Autodesk Inventor part; units mm, degrees
ref_plane "YZ Plane" through (0, 0, 0) normal (1, 0, 0) x (0, 1, 0)
ref_plane "XZ Plane" through (0, 0, 0) normal (0, 1, 0) x (-1, 0, 0)
ref_plane "XY Plane" through (0, 0, 0) normal (0, 0, 1) x (1, 0, 0)
sketch "Sketch1" plane through (0, 0, 0) normal (0, 1, 0) x (-1, 0, 0)
  line L0 (0, 0) -> (73, 0)
  line L1 (73, 0) -> (73, -56)
  line L2 (73, -56) -> (0, -56)
  line L3 (0, -56) -> (0, 0)
  dimension "d0" = 73
  dimension "d1" = 56
extrude "Extrusion1" add sketch "Sketch1" along normal blind 5
sketch "Sketch2" plane through (0, 5, 0) normal (0, 1, 0) x (1, 0, 0)
  line L0 (-73, 46) -> (-63, 46)
  line L1 (-63, 46) -> (-63, 36)
  line L2 (-63, 36) -> (-73, 36)
  line L3 (-73, 36) -> (-73, 46)
  line L4 (-10, 46) -> (0, 46)
  line L5 (0, 46) -> (0, 36)
  line L6 (0, 36) -> (-10, 36)
  line L7 (-10, 36) -> (-10, 46)
  line L8 (-73, 20) -> (-63, 20)
  line L9 (-63, 20) -> (-63, 10)
  line L10 (-63, 10) -> (-73, 10)
  line L11 (-73, 10) -> (-73, 20)
  line L12 (-10, 20) -> (0, 20)
  line L13 (0, 20) -> (0, 10)
  line L14 (0, 10) -> (-10, 10)
  line L15 (-10, 10) -> (-10, 20)
  line L16 (-73, 56) -> (-73, 0)
  line L17 (0, 0) -> (0, 56)
  line L18 (0, 56) -> (-73, 56)
  line L19 (-73, 0) -> (0, 0)
  dimension "d4" = 10
  dimension "d5" = 10
  dimension "d6" = 10
  dimension "d7" = 10
  dimension "d8" = 10
  dimension "d9" = 10
  dimension "d10" = 10
  dimension "d11" = 10
  dimension "d12" = 10
  dimension "d13" = 10
  dimension "d14" = 10
  dimension "d15" = 10
extrude "Extrusion2" add sketch "Sketch2" along normal blind 10 contours L0 L1 L2 L3 | L8 L9 L10 L11 | L5 L6 L7 L4 | L13 L14 L15 L12
hole "Hole1" at (-68, 10, -46) direction (0, 0, 1) diameter 4.3 end through all
hole "Hole2" at (-5, 10, -46) direction (0, 0, 1) diameter 4.3 end through all
sketch "Sketch4" plane through (0, 0, 0) normal (0, -1, 0) x (1, 0, 0)
  line L0 (-63.15, 19.6) -> (-9.85, 19.6)
  line L1 (-9.85, 19.6) -> (-9.85, -49)
  line L2 (-9.85, -49) -> (-63.15, -49)
  line L3 (-63.15, -49) -> (-63.15, 19.6)
  line L4 (0, -56) -> (-73, -56)
  line L5 (-73, 0) -> (-73, -56)
  circle A0 centre (-55.55, -46.5) radius 1.6
  circle A1 centre (-27.65, -46.5) radius 1.6
  circle A2 centre (-12.45, 4.3) radius 1.6
  circle A3 centre (-60.65, 5.6) radius 1.6
  point P0 (0, 0)
  dimension "d40" = 53.3
  dimension "d41" = 68.6
  dimension "d42" = 7
  dimension "d43" = 9.85
  dimension "d44" = 3.2
  dimension "d45" = 3.2
  dimension "d46" = 3.2
  dimension "d47" = 3.2
  dimension "d48" = 14
  dimension "d49" = 15.3
  dimension "d50" = 2.5
  dimension "d51" = 7.6
  dimension "d52" = 66.1
  dimension "d53" = 66.1
  dimension "d54" = 27.9
  dimension "d55" = 15.2
sketch "Sketch5" plane through (-73, 0, 0) normal (0, 0, 1) x (1, 0, 0)
  line L0 (10, 5) -> (63, 5)
  line L1 (63, 5) -> (63, 0)
  line L2 (63, 0) -> (10, 0)
  line L3 (10, 0) -> (10, 5)
  line L4 (73, 0) -> (0, 0)
  line L5 (0, 5) -> (73, 5)
  line L6 (73, 0) -> (73, 5)
  dimension "d56" = 10
  dimension "d57" = 10
extrude "Extrusion3" add sketch "Sketch5" along normal blind 10 contours L0 L1 L2 L3
extrude "Extrusion4" cut sketch "Sketch4" against normal up to next contours A0 | A1 | A2 | A3
properties part number "arduinoPlate" material "ABS Plastic"
The model under review builds one solid part; all positions refer to its coordinate system, in mm. A direction names the side the tool comes from. Round coordinates to 2 decimals unless told otherwise and drop trailing zeros. Write each loop counter-clockwise with the first axis right and the second up, starting at its lowest first coordinate (ties: lowest second). Pieces come first, ordered by that corner, then holes. Notation, with made-up numbers: M 4,55 L 14,55 A29 cw 14,88 Z; hole C -12.5,-20 d7. An arc over 180 degrees is marked long. Use a Markdown table: item, result. Add a question column.
Q1. We need section D-D, the plane z = 1.5. State the section outline as (x, y) points, plus the area to 3 significant figures.
Q2. To check wall thickness, follow line 1 (X direction, y = 10, z = -42.5); line 2 (Y direction, x = -68, z = -39.5); line 3 (X direction, y = 7.75, z = -15). State the ranges of each line that lie inside material, in increasing order.
Q3. We need section C-C, the plane y = 11.25. Count the separate pieces of the cut face and the enclosed holes in it, plus the area to 3 significant figures.
Q4. Machinability: for faces 4 (the face through (-65.7, 9.9, -36)), 5 (the face through (-65.7, 9.9, -10)), 6 (the face through (-63, 10, -41)), 7 (the face through (-63, 2, 5)), 8 (the face through (-5, 2, 0)), which of the approach directions +Z, -Z, +X, -X, +Y, -Y give a long, thin tool a straight path to every point of the face, cutting with its end or side? Answer none if there is none.
Q5. Insertion check: pin 1 (5 mm diameter, centred on x = -69.5, y = 9, fed in from -Z); pin 2 (4 mm diameter, centred on x = -12.45, z = 4.3, fed in from +Y); pin 3 (1.5 mm diameter, centred on y = 3, z = 4, fed in from -X). Each pin has a flat end and moves straight along its axis. Give the tip position at first contact, or say it passes through.
Q6. We need section B-B, the plane x = -5. State the section outline as (y, z) points, plus the area to 3 significant figures.
Q7. We need section A-A, the plane x = -12.45. State the section outline as (y, z) points.
Q8. The part is to be moulded in two halves that separate along Y. For faces 1 (the face through (-66.09, 10.99, -14.93)), 2 (the face through (-37, 3, 10)), 3 (the face through (-5, 15, -15)), say which applies: pulls with the +Y half, pulls with the -Y half, needs draft (parallel to the pull), parting line crosses it, or undercut.
Findings below:
| question | item | result |
|---|---|---|
| 1 | outline | M -63,0 L -10,0 L -10,5 L -63,5 Z |
| 1 | area | 265 mm² |
| 2 | line 1 | x = -73 to -70.15, -65.85 to -63, -10 to -7.15, -2.85 to 0 |
| 2 | line 2 | y = 0 to 7.85, 12.15 to 15 |
| 2 | line 3 | x = -73 to -63, -10 to 0 |
| 3 | separate pieces | 8 |
| 3 | enclosed holes | 0 |
| 3 | area | 260 mm² |
| 4 | face 4 | +X, -X, +Y |
| 4 | face 5 | +Z, +X, -X, +Y |
| 4 | face 6 | +Z, -Z, +Y |
| 4 | face 7 | +Z, -X, +Y, -Y |
| 4 | face 8 | +Z, +X, +Y, -Y |
| 5 | pin 1 | stops at z = -46 |
| 5 | pin 2 | stops at y = 5 |
| 5 | pin 3 | stops at x = -63 |
| 6 | outline | M 0,-56 L 5,-56 L 5,-46 L 7.85,-46 L 7.85,-36 L 5,-36 L 5,-20 L 7.85,-20 L 7.85,-10 L 5,-10 L 5,0 L 0,0 Z; M 12.15,-46 L 15,-46 L 15,-36 L 12.15,-36 Z; M 12.15,-20 L 15,-20 L 15,-10 L 12.15,-10 Z |
| 6 | area | 394 mm² |
| 7 | outline | M 0,-56 L 5,-56 L 5,2.7 L 0,2.7 Z; M 0,5.9 L 5,5.9 L 5,10 L 0,10 Z |
| 8 | face 1 | undercut |
| 8 | face 2 | needs draft |
| 8 | face 3 | pulls with the +Y half |
